Autodesk Inventor part; units mm, degrees
ref_plane "YZ Plane" through (0, 0, 0) normal (1, 0, 0) x (0, 1, 0)
ref_plane "XZ Plane" through (0, 0, 0) normal (0, 1, 0) x (-1, 0, 0)
ref_plane "XY Plane" through (0, 0, 0) normal (0, 0, 1) x (1, 0, 0)
sketch "Sketch1" plane through (0, 0, 0) normal (0, 0, 1) x (1, 0, 0)
  line L0 (-12, 12.5) -> (12, 12.5)
  line L1 (12, -12.5) -> (-12, -12.5)
  line L2 (-12, -12.5) -> (-12, 12.5)
  line L3 (-12, 12.5) -> (12, -12.5) construction
  line L4 (12, 12.5) -> (-12, -12.5) construction
  circle A0 centre (-10, 10.5) radius 1.05
  circle A1 centre (-10, -10.5) radius 1.05
  circle A2 centre (2.5, 10.5) radius 1.05
  circle A3 centre (2.5, -10.5) radius 1.05
  line L5 (12, -10.4) -> (6.5, -10.4)
  line L6 (12, 10.4) -> (6.5, 10.4)
  line L7 (6.5, 10.4) -> (6.5, -10.4)
  line L8 (12, 12.5) -> (12, 10.4)
  line L9 (12, -10.4) -> (12, -12.5)
  point P0 (0, 0)
  dimension "d0" = 24
  dimension "d1" = 25
  dimension "d2" = 2.1
  dimension "d3" = 2
  dimension "d4" = 2
  dimension "d5" = 2.1
  dimension "d6" = 2
  dimension "d7" = 2
  dimension "d8" = 2.1
  dimension "d10" = 2
  dimension "d11" = 2.1
  dimension "d12" = 2
  dimension "d14" = 5.5
  dimension "d16" = 2.1
  dimension "d17" = 2.1
  dimension "d18" = 20.8
  dimension "d19" = 9.5
  dimension "d20" = 9.5
extrude "Extrusion1" add sketch "Sketch1" along normal blind 3
equation "\"d17\" = d16"
properties part number "Camera-Holder_Camera-Base"
The model under review builds one solid part; all positions refer to its coordinate system, in mm. A direction names the side the tool comes from. Coordinates: 2 decimals unless noted, no trailing zeros. Loops run counter-clockwise (first coordinate to the right, second up) from the corner with the lowest first, then second, coordinate; pieces in that order, holes last. Notation, with made-up numbers: (-28.75, -7) -> (19.25, -7) arc R11 cw to (19.25, 9) -> close; hole circle Ø6 at (47, -7). An arc over 180 degrees is marked (long way). Answer as CSV lines item,"result".
Item 1: Take a section at C-C, the plane y = 2.25. State the section outline as (x, z) points, and give its area (3 significant figures).
Results below:
outline,"(-12, 0) -> (6.5, 0) -> (6.5, 3) -> (-12, 3) -> close"
area,"55.5 mm2"
Item 2: Take a section at A-A, the plane x = -10. State the section outline as (y, z) points.
Results below:
outline,"(-12.5, 0) -> (-11.55, 0) -> (-11.55, 3) -> (-12.5, 3) -> close; (-9.45, 0) -> (9.45, 0) -> (9.45, 3) -> (-9.45, 3) -> close; (11.55, 0) -> (12.5, 0) -> (12.5, 3) -> (11.55, 3) -> close"
Item 3: Draft analysis for pull direction Y (two halves, no side actions). For faces 3 (the cylindrical face through (-9, -10.82, 1.48)), 4 (the flat face through (0, 12.5, 1)), 5 (the cylindrical face through (-9.44, 9.61, 1.48)), 6 (the flat face through (-3, 0, 0)), state which applies: +Y half, -Y half, draft (parallel to the pull), parting line (faces both ways), or undercut.
Results below:
face 3,"undercut"
face 4,"+Y half"
face 5,"undercut"
face 6,"draft"
Item 4: Machinability: for faces 1 (the flat face through (0, -12.5, 1)), 2 (the flat face through (9, -10.4, 1)), which of the approach directions +Z, -Z, +X, -X, +Y, -Y give a long, thin tool a straight path to every point of the face, cutting with its end or side? Answer none if there is none.
Results below:
face 1,"+Z, -Z, +X, -X, -Y"
face 2,"+Z, -Z, +X"
Item 5: Insertion check: pin 1 (1.3 mm diameter, centred on x = -10, y = -10.5, fed in from +Z). The pin has a flat end and moves straight along its axis. Give the tip position at first contact, or say it passes through.
Results below:
pin 1,"passes through"
Item 6: For L1, parallel to Y at x = -10, z = 0.7; L2, parallel to Y at x = 10.25, z = 1.05; L3, parallel to X at y = -9.75, z = 0.85, list the stretches that pass through material, from the lowest coordinate up.
Results below:
L1,"y = -12.5 to -11.55, -9.45 to 9.45, 11.55 to 12.5"
L2,"y = -12.5 to -10.4, 10.4 to 12.5"
L3,"x = -12 to -10.73, -9.27 to 1.77, 3.23 to 6.5"
Item 7: Take a section at B-B, the plane z = 0.45. State the section outline as (x, y) points, and give its area (3 significant figures).
Results below:
outline,"(-12, -12.5) -> (12, -12.5) -> (12, -10.4) -> (6.5, -10.4) -> (6.5, 10.4) -> (12, 10.4) -> (12, 12.5) -> (-12, 12.5) -> close; hole circle Ø2.1 at (-10, -10.5); hole circle Ø2.1 at (-10, 10.5); hole circle Ø2.1 at (2.5, -10.5); hole circle Ø2.1 at (2.5, 10.5)"
area,"472 mm2"
